```python
from build123d import *

# Parameters (mm, degrees)
F1_DEPTH  = 45
F2_W      = 5.5
F2_H      = 2
F3_DEPTH  = 25
F5_DEPTH  = 25
F7_DEPTH  = 25
F9_DEPTH  = 5.5
F11_DEPTH = 2
F12_W     = 5
F12_H     = 14.6
F13_DEPTH = 25


with BuildPart() as f1:
    # F0 (on Top) → F1 (new body)
    with BuildSketch(Plane.XY):
        Polygon((-11.7355339059, 9.3), (-21.0355339059, 0), (-11.7355339059, -9.3), (11.7355339059, -9.3), (21.0355339059, 0), (11.7355339059, 9.3), align=None)
        Polygon((10.9071067812, -7.3), (-10.9071067812, -7.3), (-18.2071067812, 0), (-10.9071067812, 7.3), (10.9071067812, 7.3), (18.2071067812, 0), align=None, mode=Mode.SUBTRACT)
    extrude(amount=F1_DEPTH)

    # F2 (on face) → F3 (cut)
    with BuildSketch(Plane.XY.offset(45)):
        with Locations((0, 8.3)):
            Rectangle(F2_W, F2_H)
    extrude(amount=-F3_DEPTH, mode=Mode.SUBTRACT)

    # F4 (on face) → F5 (join)
    with BuildSketch(Plane.XY.offset(45)):
        Polygon((2.75, 11.3), (2.75, 9.3), (4.75, 9.3), (4.75, 13.3), (-4.75, 13.3), (-4.75, 9.3), (-2.75, 9.3), (-2.75, 11.3), align=None)
    extrude(amount=-F5_DEPTH)

    # F6 (on face) → F7 (cut)
    with BuildSketch(Plane.YZ.offset(4.75)):
        Polygon((13.3, 26.9282032303), (9.3, 20), (13.3, 20), align=None)
    extrude(amount=-F7_DEPTH, mode=Mode.SUBTRACT)

    # F8 (on face) → F9 (join, through all)
    with BuildSketch(Plane.YZ.offset(-2.75)):
        Polygon((7.3, 20), (9.3, 20), (11.3, 23.4641016151), (11.3, 26.9282032303), align=None)
    extrude(amount=F9_DEPTH)

    # F10 (on face) → F11 (join)
    with BuildSketch(Plane(origin=(0, 0, 0), x_dir=(1, 0, 0), z_dir=(0, 0, -1))):
        Polygon((-11.7355339059, 9.3), (-21.0355339059, 0), (-11.7355339059, -9.3), (11.7355339059, -9.3), (21.0355339059, 0), (11.7355339059, 9.3), align=None)
        Polygon((-18.2071067812, 0), (-10.9071067812, 7.3), (10.9071067812, 7.3), (18.2071067812, 0), (10.9071067812, -7.3), (-10.9071067812, -7.3), align=None, mode=Mode.SUBTRACT)
        Polygon((10.9071067812, 7.3), (-10.9071067812, 7.3), (-18.2071067812, 0), (-10.9071067812, -7.3), (10.9071067812, -7.3), (18.2071067812, 0), align=None)
    extrude(amount=F11_DEPTH)

    # F12 (on face) → F13 (join)
    with BuildSketch(Plane.XY):
        Polygon((18.2071067812, 0), (13.2071067812, 5), (13.2071067812, -5), align=None)
        Polygon((-13.2071067812, -5), (-13.2071067812, 5), (-18.2071067812, 0), align=None)
        Rectangle(F12_W, F12_H)
    extrude(amount=F13_DEPTH)


solid = f1.part
```
Geometry: final body of the model. Coordinates: model frame, mm. A direction names the side the tool comes from. Coordinates: 2 decimals unless noted, no trailing zeros. Write each loop counter-clockwise with the first axis right and the second up, starting at its lowest first coordinate (ties: lowest second). Pieces come first, ordered by that corner, then holes. Notation, with made-up numbers: M 89,-4.75 L 108,-4.75 A24 cw 108,12.25 Z; hole C -36.75,61.5 d6. An arc over 180 degrees is marked long. Answer as CSV lines item,"result". Start each with the question number.
Q1. Reachability of faces 1 (the flat face through (-4.75, 11, 35)), 2 (the flat face through (-13.695, -4.512, 27.185)), 3 (the flat face through (0, -9.3, 22)), 4 (the flat face through (-16.32, -4.715, 21.829)), 5 (the flat face through (4.75, 11, 35)) from +Z, -Z, +X, -X, +Y, -Y: full face, straight path, thin tool, end or side. Return the list, or none.
Q2. Mould query, pull axis X, two halves, no side actions, for faces 6 (the flat face through (0, 0, -2)), 7 (the flat face through (7, 7.3, 22)), 8 (the flat face through (16.451, -4.585, 21.829)). Classes: released by +X, released by -X, zero draft, split by the parting line, or undercut.
Q3. Pin query (flat end, axial travel): P1, Ø5, axis at y = 9.5, z = 3.5, coming from the +X side; P2, Ø4, axis at x = 0, z = 23, coming from the +Y side; P3, Ø5, axis at x = 11, z = 28.5, coming from the +Y side; P4, Ø1, axis at x = 14, y = 9.5, coming from the -Z side. Return the tip coordinate at first contact, or that it passes through.
Q4. Cut plane C-C on z = 42.5. Return the cut outline in (x, y), then the cut area to 3 significant figures.
Q5. Cut plane B-B on x = -6. Return the cut outline in (y, z).
Q6. Cut plane D-D on y = -6. Return the cut outline in (x, z).
Q7. Cut plane A-A on z = 5. Return the cut outline in (x, y).
Q8. Line query: line 1 (X direction, y = 3.25, z = 13); line 2 (X direction, y = -6.75, z = 23); line 3 (Y direction, x = -4.5, z = 43.5). Output: solid intervals per line, ascending. Write a range as from..to.
Findings below:
1,face 1,"+Z, -Z, -X, +Y"
1,face 2,"+Z"
1,face 3,"+Z, -Z, +X, -X, -Y"
1,face 4,"+Z, -Z, -X, -Y"
1,face 5,"+Z, -Z, +X, +Y"
2,face 6,"zero draft"
2,face 7,"undercut"
2,face 8,"released by +X"
3,P1,"stops at x = 14.04"
3,P2,"stops at y = 12.19"
3,P3,"stops at y = 9.3"
3,P4,"passes through"
4,outline,"M -21.04,0 L -11.74,-9.3 L 11.74,-9.3 L 21.04,0 L 11.74,9.3 L 4.75,9.3 L 4.75,13.3 L -4.75,13.3 L -4.75,9.3 L -11.74,9.3 Z; hole M -18.21,0 L -10.91,-7.3 L 10.91,-7.3 L 18.21,0 L 10.91,7.3 L 2.75,7.3 L 2.75,11.3 L -2.75,11.3 L -2.75,7.3 L -10.91,7.3 Z"
4,area,"200 mm2"
5,outline,"M -9.3,-2 L 9.3,-2 L 9.3,45 L 7.3,45 L 7.3,0 L -7.3,0 L -7.3,45 L -9.3,45 Z"
6,outline,"M -15.04,-2 L 15.04,-2 L 15.04,45 L 12.21,45 L 12.21,0 L 2.5,0 L 2.5,25 L -2.5,25 L -2.5,0 L -12.21,0 L -12.21,45 L -15.04,45 Z"
7,outline,"M -21.04,0 L -11.74,-9.3 L 11.74,-9.3 L 21.04,0 L 11.74,9.3 L -11.74,9.3 Z; hole M -13.21,-5 L -10.91,-7.3 L -2.5,-7.3 L -2.5,7.3 L -10.91,7.3 L -13.21,5 Z; hole M 2.5,-7.3 L 10.91,-7.3 L 13.21,-5 L 13.21,5 L 10.91,7.3 L 2.5,7.3 Z"
8,line 1,"x = -17.79..-13.21, -2.5..2.5, 13.21..17.79"
8,line 2,"x = -14.29..-11.46, -2.5..2.5, 11.46..14.29"
8,line 3,"y = -9.3..-7.3, 7.3..13.3"
